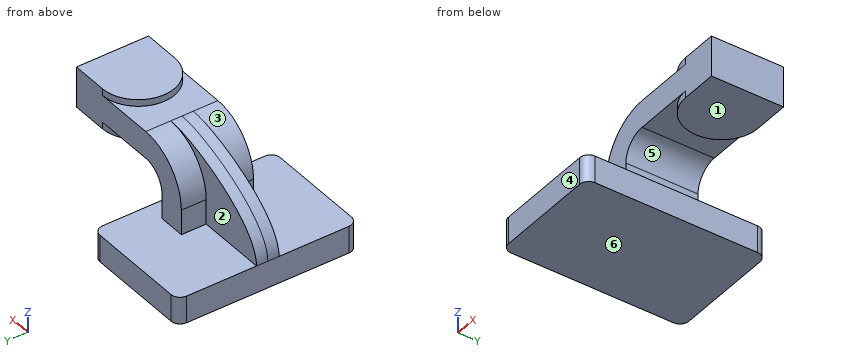
```python
from build123d import *

# Parameters (mm, degrees)
F1_DEPTH = 63.5
F0_W     = 25.4
F0_H     = 19.05
F2_DEPTH = 25.4
F3_DEPTH = 7.9375
F5_R     = 6.35


with BuildPart() as f1:
    # F0 (on Front) → F1 (new body, symmetric)
    with BuildSketch(Plane.XZ):
        Polygon((8.1319350704, 9.525), (-41.275, 9.525), (-41.275, -9.525), (41.275, -9.525), (41.275, 9.525), (27.1819350704, 9.525), align=None)
    extrude(amount=F1_DEPTH, both=True)

    # F0 (on Front) → F2 (join, symmetric)
    with BuildSketch(Plane.XZ):
        with BuildLine():
            Line((8.1319350704, 27.0002), (8.1319350704, 9.525))
            Line((8.1319350704, 9.525), (27.1819350704, 9.525))
            Line((27.1819350704, 9.525), (27.1819350704, 27.0002))
            ThreePointArc((27.1819350704, 27.0002), (31.8316149191, 38.2255201513), (43.0569350704, 42.8752))
            Line((43.0569350704, 42.8752), (60.325, 42.8752))
            Line((60.325, 42.8752), (60.325, 61.9252))
            Line((60.325, 61.9252), (43.0569350704, 61.9252))
            ThreePointArc((43.0569350704, 61.9252), (18.3612307375, 51.6959043329), (8.1319350704, 27.0002))
        make_face()
        Polygon((85.725, 66.675), (85.725, 61.9252), (85.725, 42.8752), (85.725, 38.1), (111.125, 38.1), (111.125, 66.675), align=None)
        with Locations((73.025, 52.4002)):
            Rectangle(F0_W, F0_H)
    extrude(amount=F2_DEPTH, both=True)

    # F0 (on Front) → F3 (join, symmetric)
    with BuildSketch(Plane.XZ):
        with BuildLine():
            add(Edge.make_bspline(
                [(-41.275, 9.525), (-40.8404879272, 39.9630628526), (24.2341663688, 63.2040128112), (43.0569350704, 61.9252)],
                knots=[0, 0, 0, 0, 99.2857302575, 99.2857302575, 99.2857302575, 99.2857302575], degree=3))
            Line((-41.275, 9.525), (8.1319350704, 9.525))
            Line((8.1319350704, 9.525), (8.1319350704, 27.0002))
            ThreePointArc((8.1319350704, 27.0002), (18.3612307375, 51.6959043329), (43.0569350704, 61.9252))
        make_face()
    extrude(amount=F3_DEPTH, both=True)

    # F0 (on Front) → F4 (revolve)
    with BuildSketch(Plane.XZ):
        Polygon((85.725, 66.675), (85.725, 61.9252), (85.725, 42.8752), (85.725, 38.1), (111.125, 38.1), (111.125, 66.675), align=None)
    revolve(axis=Axis((85.725, 0, 52.3875), (0, 0, 1)))

    # F5
    f5_edges = [f1.edges().sort_by_distance(p)[0] for p in [
        (-41.275, -63.5, 0),
        (41.275, -63.5, 0),
        (41.275, 63.5, 0),
        (-41.275, 63.5, 0),
    ]]
    fillet(f5_edges, radius=F5_R)


solid = f1.part
```
CAD build for the part. Positions are in the model's coordinates, mm. Face numbers are marked on the shaded views. A direction names the side the tool comes from. Coordinates: 2 decimals unless noted, no trailing zeros. Order: outer loops, then holes, each group sorted by start corner. A loop starts at its lowest first (then second) coordinate and runs counter-clockwise, first axis right, second up. Notation, with made-up numbers: (52.25, -22.75) - (76.25, -22.75) arc R3 cw to (76.25, -18.75) - close; hole circle Ø4 at (-24, 2). An arc over 180 degrees is marked (long way). Use a Markdown table: item, result. Add a question column.
(1) Flat gauge pins, fed straight in: pin 1 (14 mm diameter, centred on y = 18.5, z = 22, fed in from -X); pin 2 (1.5 mm diameter, centred on x = 25, y = 40.5, fed in from +Z) (3 decimals); pin 3 (2 mm diameter, centred on y = 3.5, z = 34, fed in from -X). Where does each tip first touch, or does it go through?
(2) Which spindle directions (+Z, -Z, +X, -X, +Y, -Y) get a long thin tool onto all of the face, cutting with end or side? Do the marked faces 1, 2 and 3. Say none if no direction does.
(3) Saw through at A-A (z = -0.5). Give the cut face in (x, y) (3 decimals), then the cut area to 3 significant figures.
(4) Drill centre lines: line 1 along Z through (x, y) = (-19.5, -24) (3 decimals); line 2 along Y through (x, z) = (-25, 19); line 3 along Y through (x, z) = (20.5, 30). Where is each one in solid material? Low to high. Write a range as [from, to].
(5) Saw through at C-C (x = 47). Give the cut face in (y, z), then the cut area to 3 significant figures.
(6) Saw through at D-D (y = -38). Give the cut face in (x, z) (3 decimals).
(7) Pull direction Z, two halves, no side cores. Call the marked faces 4, 5 and 6: +Z half, -Z half, draft (parallel to the pull), parting line (faces both ways), or undercut.
(8) Saw through at B-B (y = 18). Give the cut face in (x, z) (3 decimals), then the cut area to 3 significant figures.
Solved:
| question | item | result |
|---|---|---|
| 1 | pin 1 | stops at x = 8.13 |
| 1 | pin 2 | stops at z = 9.525 |
| 1 | pin 3 | stops at x = -28.16 |
| 2 | face 1 | -Z, +X, +Y, -Y |
| 2 | face 2 | +Z, -X, +Y |
| 2 | face 3 | +Z, -X, -Y |
| 3 | outline | (-41.275, -57.15) arc R6.35 ccw to (-34.925, -63.5) - (34.925, -63.5) arc R6.35 ccw to (41.275, -57.15) - (41.275, 57.15) arc R6.35 ccw to (34.925, 63.5) - (-34.925, 63.5) arc R6.35 ccw to (-41.275, 57.15) - close |
| 3 | area | 10,400 mm² |
| 4 | line 1 | z = [-9.525, 9.525] |
| 4 | line 2 | y = [-7.94, 7.94] |
| 4 | line 3 | y = [-25.4, 25.4] |
| 5 | outline | (-25.4, 42.88) - (25.4, 42.88) - (25.4, 61.93) - (-25.4, 61.93) - close |
| 5 | area | 968 mm² |
| 6 | outline | (-41.275, -9.525) - (41.275, -9.525) - (41.275, 9.525) - (-41.275, 9.525) - close |
| 7 | face 4 | draft |
| 7 | face 5 | undercut |
| 7 | face 6 | -Z half |
| 8 | outline | (-41.275, -9.525) - (41.275, -9.525) - (41.275, 9.525) - (27.182, 9.525) - (27.182, 27) arc R15.875 cw to (43.057, 42.875) - (67.804, 42.875) - (67.804, 38.1) - (111.125, 38.1) - (111.125, 66.675) - (67.804, 66.675) - (67.804, 61.925) - (43.057, 61.925) arc R34.925 ccw to (8.132, 27) - (8.132, 9.525) - (-41.275, 9.525) - close |
| 8 | area | 4,370 mm² |
